```python
from build123d import *

# Parameters (mm, degrees)
F0_R     = 5
F1_DEPTH = 15
F0_R_2   = 12
F2_DEPTH = 30


with BuildPart() as f1:
    # F0 (on Top) → F1 (new body)
    with BuildSketch(Plane.XY):
        with BuildLine():
            ThreePointArc((5, 19.364917), (15.811388, 12.247449), (20, 0))
            ThreePointArc((20, 0), (15.811388, -12.247449), (5, -19.364917))
            Line((5, -19.364917), (42.5, -9.682458))
            ThreePointArc((42.5, -9.682458), (50, 0), (42.5, 9.682458))
            Line((42.5, 9.682458), (5, 19.364917))
        make_face()
        with Locations((40, 0)):
            Circle(F0_R, mode=Mode.SUBTRACT)
    extrude(amount=F1_DEPTH)

    # F0 (on Top) → F2 (join)
    with BuildSketch(Plane.XY):
        with BuildLine():
            ThreePointArc((5, -19.364917), (15.811388, -12.247449), (20, 0))
            ThreePointArc((20, 0), (15.811388, 12.247449), (5, 19.364917))
            ThreePointArc((5, 19.364917), (-19.989625, 0.644109), (3.742964, -19.646634))
            Line((3.742964, -19.646634), (5, -19.364917))
        make_face()
        Circle(F0_R_2, mode=Mode.SUBTRACT)
    extrude(amount=F2_DEPTH)


solid = f1.part
```
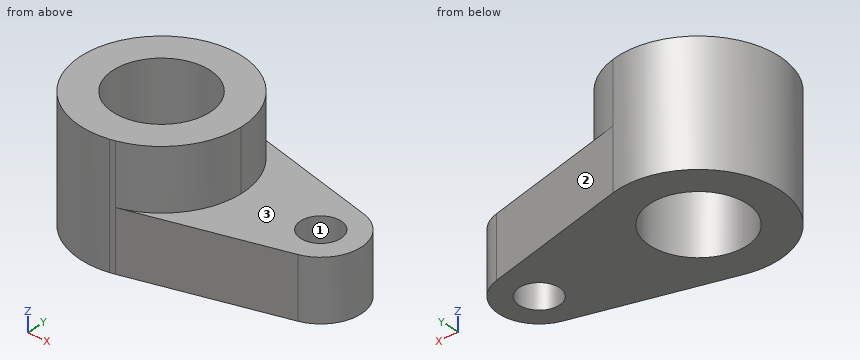
Geometry check sheet. Reference: the model listing, model coordinates, mm. Face numbers are marked on the shaded views. Coordinates: 2 decimals unless noted, no trailing zeros. Write each loop counter-clockwise with the first axis right and the second up, starting at its lowest first coordinate (ties: lowest second). Pieces come first, ordered by that corner, then holes. Notation, with made-up numbers: M 35,-30 L 42,-30 A9 ccw 42,-21 Z; hole C 64.25,77.5 d8. An arc over 180 degrees is marked long. Answer as a JSON object with one key per item and string values.
1. Section check A-A, the plane x = 0. Enter the section's corners in (y, z).
Answers below:
{"outline": "M -20,0 L -12,0 L -12,30 L -20,30 Z; M 12,0 L 20,0 L 20,30 L 12,30 Z"}
2. Draft check along X on the marked faces 1, 2 and 3. Enter one of: released by +X, released by -X, zero draft, split by the parting line, or undercut.
Answers below:
{"face 1": "undercut", "face 2": "released by +X", "face 3": "zero draft"}
3. Section check C-C, the plane z = 27.5. Enter the section's corners in (x, y).
Answers below:
{"outline": "M 3.74,-19.65 L 5,-19.36 A20 ccw 5,19.36 A20 ccw long Z; hole C 0,0 d24"}
4. Section check B-B, the plane z = 6.75. Enter the section's corners in (x, y).
Answers below:
{"outline": "M 3.74,-19.65 L 5,-19.36 L 42.5,-9.68 A10 ccw 42.5,9.68 L 5,19.36 A20 ccw long Z; hole C 0,0 d24; hole C 40,0 d10"}
5. Go/stop test with flat-tipped pins: pin 1 Ø10 at (x, z) = (-9, 20) entering from -Y; pin 2 Ø8 at (y, z) = (8, 11.5) entering from -X; pin 3 Ø5 at (x, y) = (22.5, -1.5) entering from +Z. Record where each tip stops, or that it passes through.
Answers below:
{"pin 1": "stops at y = -19.6", "pin 2": "stops at x = -19.6", "pin 3": "stops at z = 15"}
6. Scan lines: L1, parallel to X at y = -7, z = 15.5 (3 decimals); L2, parallel to X at y = -7.5, z = 21.5; L3, parallel to Y at x = -5, z = 6.75. Record each from-to range of solid material in increasing order.
Answers below:
{"L1": "x = -18.735 to -9.747, 9.747 to 18.735", "L2": "x = -18.54 to -9.37, 9.37 to 18.54", "L3": "y = -19.36 to -10.91, 10.91 to 19.36"}
7. Section check D-D, the plane y = 6.5. Enter the section's corners in (x, z), plus the area to 3 significant figures.
Answers below:
{"outline": "M -18.91,0 L -10.09,0 L -10.09,30 L -18.91,30 Z; M 10.09,0 L 47.6,0 L 47.6,15 L 18.91,15 L 18.91,30 L 10.09,30 Z", "area": "960 mm²"}
